Read the model definition and answer for the solid it produces. Units are mm, in the model's axes. A direction names the side the tool comes from. Round coordinates to 2 decimals unless told otherwise and drop trailing zeros. Loops run counter-clockwise (first coordinate to the right, second up) from the corner with the lowest first, then second, coordinate; pieces in that order, holes last. Notation, with made-up numbers: M -38.75,-4.75 L -8.75,-4.75 A25 cw -8.75,32.25 Z; hole C 23,-3.5 d10. An arc over 180 degrees is marked long. Write each question's results on one line, items separated by ' | '.
from build123d import *

# Parameters (mm, degrees)
SKETCH1_R               = 16.892448346
BOSS_EXTRUDE1_DEPTH     = 70
SKETCH2_W               = 51.249127752
SKETCH2_H               = 51.249127751
BOSS_EXTRUDE2_DEPTH     = 10
CUT_EXTRUDE1_DEPTH      = 20.696737014
CUT_EXTRUDE1_DEPTH_BACK = 32.552390737


with BuildPart() as part:
    # Sketch1 → Boss-Extrude1 (new body)
    with BuildSketch(Plane.XY):
        with Locations((-8.123318292, -5.927826862)):
            Circle(SKETCH1_R)
    extrude(amount=BOSS_EXTRUDE1_DEPTH)

    # Sketch2 → Boss-Extrude2 (add)
    with BuildSketch(Plane.XY.offset(70)):
        with Locations((-8.123318292, -5.927826862)):
            Rectangle(SKETCH2_W, SKETCH2_H)
    extrude(amount=BOSS_EXTRUDE2_DEPTH)

    # Sketch3 → Cut-Extrude1 (cut, two sides)
    with BuildSketch(Plane(origin=(0, 0, 0), x_dir=(1, 0, 0), z_dir=(0, 1, 0))) as cut_extrude1_sk:
        Polygon((-25.712291526, 12.946943155), (18.961130043, -104.420154992), (40.320792226, 8.610459854), align=None)
    extrude(amount=CUT_EXTRUDE1_DEPTH, mode=Mode.SUBTRACT)
    extrude(cut_extrude1_sk.sketch, amount=-CUT_EXTRUDE1_DEPTH_BACK, mode=Mode.SUBTRACT)


solid = part.part
Item 1: Flat-ended cylindrical pins translate along their axes: pin 1 (10 mm diameter, centred on y = -24, z = 37.5, fed in from +X); pin 2 (3 mm diameter, centred on x = -17, z = 62, fed in from +Y); pin 3 (8 mm diameter, centred on y = -1, z = 41, fed in from +X). Find the tip coordinate at first contact, or state that the pin passes through.
Outcome:
pin 1: stops at x = -4.7 | pin 2: stops at y = 9.27 | pin 3: stops at x = -3.66
Item 2: The part is cut by section C-C (z = 59). Determine the outline of the cut face in (x, y).
Outcome:
outline: M 1.67,-19.69 L 1.67,7.83 A16.89 ccw long Z
Item 3: The part is cut by section D-D (y = 16). Determine the outline of the cut face in (x, z).
Outcome:
outline: M -33.75,70 L 5.86,70 L 9.67,80 L -33.75,80 Z
Item 4: The part is cut by section B-B (y = -21). Determine the outline of the cut face in (x, z).
Outcome:
outline: M -33.75,70 L -15.75,70 L -15.75,13.22 L -0.5,53.3 L -0.5,70 L 5.86,70 L 9.67,80 L -33.75,80 Z
Item 5: Straight lines are drawn through the part: line 1 (Z direction, x = -32, y = 12.5); line 2 (Y direction, x = -15.5, z = 40); line 3 (X direction, y = 3, z = 41). For each, find the intervals that lie inside material, in ascending order.
Outcome:
line 1: z = 70 to 80 | line 2: y = -21.12 to 9.27 | line 3: x = -22.46 to -5.18
Item 6: The part is cut by section A-A (x = -11). Determine the outline of the cut face in (y, z), plus the area to 3 significant figures.
Outcome:
outline: M -31.55,70 L -22.57,70 L -22.57,25.71 L 10.72,25.71 L 10.72,70 L 19.7,70 L 19.7,80 L -31.55,80 Z | area: 1,990 mm2
Item 7: For faces 1 (the face through (-25.005, -5.326, 42.288)), 2 (the face through (-5.772, -5.569, 39.44)), determine the directions among +Z, -Z, +X, -X, +Y, -Y from which every point of the face is accessible in a straight line to the end or side of a thin tool.
Outcome:
face 1: -Z | face 2: -Z, +X, +Y, -Y
